Autodesk Inventor part; units mm, degrees
ref_plane "YZ Plane" through (0, 0, 0) normal (1, 0, 0) x (0, 1, 0)
ref_plane "XZ Plane" through (0, 0, 0) normal (0, 1, 0) x (-1, 0, 0)
ref_plane "XY Plane" through (0, 0, 0) normal (0, 0, 1) x (1, 0, 0)
sketch "Sketch1" plane through (0, 0, 0) normal (0, 0, 1) x (1, 0, 0)
  line L0 (151.8583, 166.9217) -> (156.9383, 166.9217)
  line L1 (156.9383, 166.9217) -> (156.9383, 161.8417)
  line L2 (156.9383, -10.8783) -> (-20.8617, -10.8783)
  line L3 (-20.8617, -10.8783) -> (-20.8617, 166.9217)
  line L4 (-20.8617, -5.7983) -> (151.8583, 166.9217)
  line L5 (-15.7817, -10.8783) -> (156.9383, 161.8417)
  point P0 (0, 0)
  dimension "d0" = 177.8
  dimension "d1" = 177.8
  dimension "d2" = 45
  dimension "d3" = 45
  dimension "d4" = 5.08
  dimension "d5" = 5.08
extrude "Extrusion1" add sketch "Sketch1" along normal blind 177.8
properties part number "Redirection Plate"
For this review, take the finished solid that the model builds, in its own axes (mm). Give positions to 0.01 mm unless a question says otherwise; leave off trailing zeros. Order: outer loops, then holes, each group sorted by start corner. A loop starts at its lowest first (then second) coordinate and runs counter-clockwise, first axis right, second up.
1) Take a section at B-B (x = 50). Give the boundary of the cut face in (y, z).
2) Wall thickness on line 1 (X direction, y = 129, z = 151.5); line 2 (X direction, y = 119, z = 137); line 3 (Y direction, x = 141.5, z = 119.5): over which ranges is each line inside the solid? List them lowest first.
3) Take a section at A-A (z = 17.5). Give the boundary of the cut face in (x, y), then the cut area to 3 significant figures.
4) Insertion check: pin 1 (8 mm diameter, centred on x = 28.5, z = 102.5, fed in from -Y); pin 2 (5 mm diameter, centred on y = 45.5, z = 84, fed in from -X); pin 3 (2 mm diameter, centred on y = 118, z = 134, fed in from -X); pin 4 (1 mm diameter, centred on x = 80.5, y = 86, fed in from -Z). Each pin has a flat end and moves straight along its axis. Give the tip position at first contact, or say it passes through.
5) Take a section at C-C (y = 116). Give the boundary of the cut face in (x, z), then the cut area to 3 significant figures.
Derived:
1. outline: (54.9, 0) - (65.06, 0) - (65.06, 177.8) - (54.9, 177.8) - close
2. line 1: x = 113.94 to 124.1
2. line 2: x = 103.94 to 114.1
2. line 3: y = 146.4 to 156.56
3. outline: (-20.86, -10.88) - (-15.78, -10.88) - (156.94, 161.84) - (156.94, 166.92) - (151.86, 166.92) - (-20.86, -5.8) - close
3. area: 1,780 mm2
4. pin 1: stops at y = 29.4
4. pin 2: stops at x = 27.94
4. pin 3: stops at x = 101.94
4. pin 4: stops at z = 0
5. outline: (100.94, 0) - (111.1, 0) - (111.1, 177.8) - (100.94, 177.8) - close
5. area: 1,810 mm2
